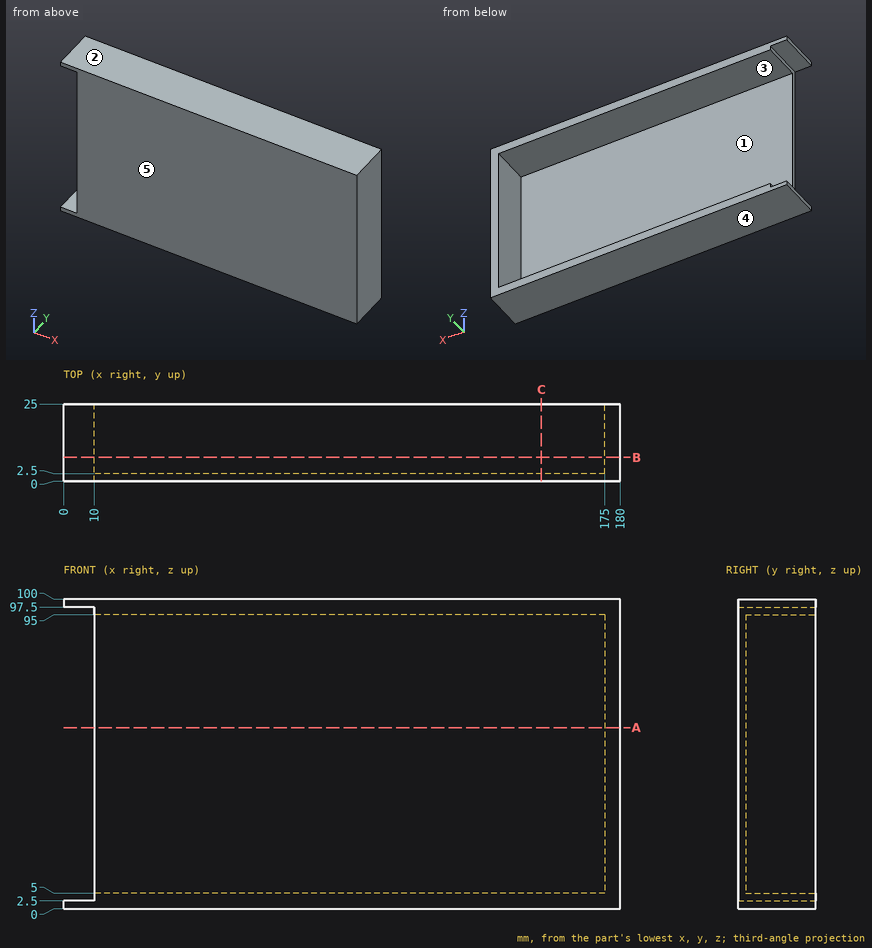
The drawing under review shows one solid part. Ordinate dimensions are in mm from its lowest x, y, z. A direction names the side the tool comes from. Coordinates: 2 decimals unless noted, no trailing zeros. Write each loop counter-clockwise with the first axis right and the second up, starting at its lowest first coordinate (ties: lowest second). Pieces come first, ordered by that corner, then holes.
1) Machinability: for the marked faces 1 and 2, which of the approach directions +Z, -Z, +X, -X, +Y, -Y give a long, thin tool a straight path to every point of the face, cutting with its end or side? Answer none if there is none.
2) Add section B-B (y = 7.75). Write out the cut boundary in (x, z), plus the area to 3 significant figures.
3) Insertion check: pin 1 (10 mm diameter, centred on x = 80, z = 39.5, fed in from +Y); pin 2 (8 mm diameter, centred on y = 17.5, z = 44, fed in from -X). Each pin has a flat end and moves straight along its axis. Give the tip position at first contact, or say it passes through.
4) Mouldability with a two-part tool opening along Z and no side actions: class the marked faces 3, 4 and 5 as +Z half, -Z half, draft (parallel to the pull), parting line (faces both ways), or undercut.
5) Add section C-C (x = 154.5). Write out the cut boundary in (y, z).
6) To check wall thickness, follow L1, parallel to Z at x = 85, y = 15.25; L2, parallel to Y at x = 116.5, z = 69.5; L3, parallel to X at y = 23.75, z = 12. State the ranges of each line that lie inside material, in increasing order.
7) Add section A-A (z = 58.5). Write out the cut boundary in (x, y), plus the area to 4 significant figures.
Check result:
1. face 1: -X, +Y
1. face 2: +Z, +X, -X, +Y, -Y
2. outline: (0, 0) - (180, 0) - (180, 100) - (0, 100) - (0, 97.5) - (10, 97.5) - (10, 95) - (175, 95) - (175, 5) - (10, 5) - (10, 2.5) - (0, 2.5) - close
2. area: 2,200 mm2
3. pin 1: stops at y = 2.5
3. pin 2: stops at x = 175
4. face 3: undercut
4. face 4: -Z half
4. face 5: draft
5. outline: (0, 0) - (25, 0) - (25, 5) - (2.5, 5) - (2.5, 95) - (25, 95) - (25, 100) - (0, 100) - close
6. L1: z = 0 to 5, 95 to 100
6. L2: y = 0 to 2.5
6. L3: x = 175 to 180
7. outline: (10, 0) - (180, 0) - (180, 25) - (175, 25) - (175, 2.5) - (10, 2.5) - close
7. area: 537.5 mm2
